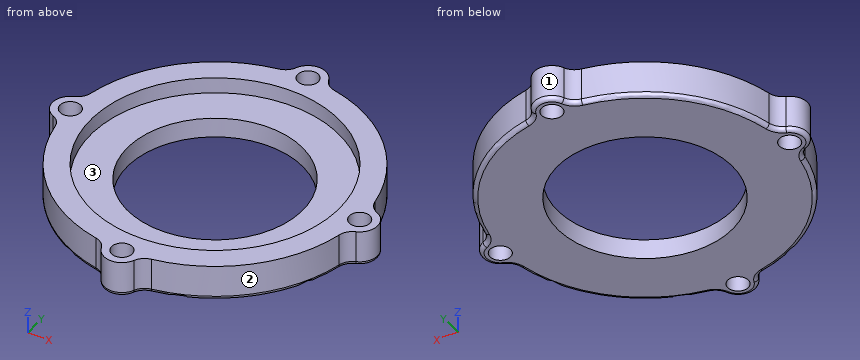
```python
from build123d import *

# Parameters (mm, degrees)
SKETCH_R      = 22
SKETCH_R_2    = 2.6
PAD_DEPTH     = 9
SKETCH001_R   = 31.2
SKETCH001_R_2 = 22
POCKET_DEPTH  = 4
FILLET_R      = 4
FILLET001_R   = 1


with BuildPart() as part:
    # Sketch → Pad (new body)
    with BuildSketch(Plane.XY):
        with BuildLine():
            ThreePointArc((-4.5, 36.725332), (-26.162951, 26.162951), (-36.725332, 4.5))
            Line((-37.000025, 4.5), (-36.725332, 4.5))
            ThreePointArc((-37.000025, 4.5), (-41.5, 0), (-37.000025, -4.5))
            Line((-37.000025, -4.5), (-36.725332, -4.5))
            ThreePointArc((-36.725332, -4.5), (-26.162951, -26.162951), (-4.5, -36.725332))
            Line((-4.5, -36.725332), (-4.5, -37))
            ThreePointArc((-4.5, -37), (0, -41.5), (4.5, -37.000001))
            Line((4.5, -36.725332), (4.5, -37.000001))
            ThreePointArc((4.5, -36.725332), (26.162951, -26.162951), (36.725332, -4.5))
            Line((36.725332, -4.5), (37.000003, -4.5))
            ThreePointArc((37.000003, -4.5), (41.5, 0), (37.000003, 4.5))
            Line((36.725332, 4.5), (37.000003, 4.5))
            ThreePointArc((36.725332, 4.5), (26.162951, 26.162951), (4.5, 36.725332))
            Line((4.5, 36.999999), (4.5, 36.725332))
            ThreePointArc((4.5, 36.999999), (1.1e-05, 41.5), (-4.5, 37.000021))
            Line((-4.5, 37.000021), (-4.5, 36.725332))
        make_face()
        Circle(SKETCH_R, mode=Mode.SUBTRACT)
        with Locations((0, 37)):
            Circle(SKETCH_R_2, mode=Mode.SUBTRACT)
        with Locations((0, -37)):
            Circle(SKETCH_R_2, mode=Mode.SUBTRACT)
        with Locations((-37, 0)):
            Circle(SKETCH_R_2, mode=Mode.SUBTRACT)
        with Locations((37, 0)):
            Circle(SKETCH_R_2, mode=Mode.SUBTRACT)
    extrude(amount=PAD_DEPTH)

    # Sketch001 → Pocket (cut)
    with BuildSketch(Plane.XY.offset(9)):
        Circle(SKETCH001_R)
        Circle(SKETCH001_R_2, mode=Mode.SUBTRACT)
    extrude(amount=-POCKET_DEPTH, mode=Mode.SUBTRACT)

    # Fillet
    fillet_edges = [part.edges().sort_by_distance(p)[0] for p in [
        (-36.725332, 4.5, 4.5),
        (-4.5, 36.725332, 4.5),
        (4.5, 36.725332, 4.5),
        (36.725332, 4.5, 4.5),
        (36.725332, -4.5, 4.5),
        (4.5, -36.725332, 4.5),
        (-4.5, -36.725332, 4.5),
        (-36.725332, -4.5, 4.5),
    ]]
    fillet(fillet_edges, radius=FILLET_R)

    # Fillet001
    fillet001_edges = [part.edges().sort_by_distance(p)[0] for p in [
        (-5.323601, 37.145487, 0),
        (-26.162951, 26.162951, 0),
        (0, 41.5, 0),
        (5.323601, 37.145487, 0),
        (26.162951, 26.162951, 0),
        (37.145487, 5.323601, 0),
        (41.5, 0, 0),
        (37.145487, -5.323601, 0),
        (26.162951, -26.162951, 0),
        (5.323601, -37.145487, 0),
        (0, -41.5, 0),
        (-5.323601, -37.145487, 0),
        (-26.162951, -26.162951, 0),
        (-37.145487, -5.323601, 0),
        (-41.5, 0, 0),
        (-37.145487, 5.323601, 0),
    ]]
    fillet(fillet001_edges, radius=FILLET001_R)


solid = part.part
```
Here's how the part is built. I have some questions about the finished solid (model axes, mm). Face numbers are marked on the shaded views. Round coordinates to 2 decimals unless told otherwise and drop trailing zeros. Order: outer loops, then holes, each group sorted by start corner. A loop starts at its lowest first (then second) coordinate and runs counter-clockwise, first axis right, second up. Notation, with made-up numbers: M 26.25,-23.5 L 76.25,-23.5 A25 cw 76.25,7.5 Z; hole C 29.25,3.25 d8. An arc over 180 degrees is marked long. Use CSV: the item, a comma, the result in double quotes.
1) If we mould it in two halves opening along Y, with no side actions, what happens to the marked faces 1, 2 and 3? For each: pulls with the +Y half, pulls with the -Y half, needs draft (parallel to the pull), parting line crosses it, or undercut.
Taken from the geometry:
face 1,"pulls with the +Y half"
face 2,"pulls with the -Y half"
face 3,"undercut"
2) I need wall thicknesses on line 1 along Y through (x, z) = (0, 4.5); line 2 along Y through (x, z) = (0, 6.8); line 3 along X through (y, z) = (2, 4.25). Which ranges of each line are inside material? Lowest first, please. Write a range as [from, to].
Taken from the geometry:
line 1,"[-41.5, -39.6], [-34.4, -22], [22, 34.4], [39.6, 41.5]"
line 2,"[-41.5, -39.6], [-34.4, -31.2], [31.2, 34.4], [39.6, 41.5]"
line 3,"[-41.03, -38.66], [-35.34, -21.91], [21.91, 35.34], [38.66, 41.03]"
3) I want a section at A-A (y = 0). List the corners of the cut face in (x, z) for me, then the cut area to 3 significant figures.
Taken from the geometry:
outline,"M -41.5,1 A1 ccw -40.5,0 L -39.6,0 L -39.6,9 L -41.5,9 Z; M -34.4,0 L -22,0 L -22,5 L -31.2,5 L -31.2,9 L -34.4,9 Z; M 22,0 L 34.4,0 L 34.4,9 L 31.2,9 L 31.2,5 L 22,5 Z; M 39.6,0 L 40.5,0 A1 ccw 41.5,1 L 41.5,9 L 39.6,9 Z"
area,"183 mm^2"
4) I want a section at B-B (z = 3.5). Count the separate pieces of the cut face and the enclosed holes in it, then the cut area to 3 significant figures.
Taken from the geometry:
separate pieces,"1"
enclosed holes,"5"
area,"2,830 mm^2"
5) I'm going to push flat-ended pins straight in: P1, Ø10, axis at x = 18, y = -8.5, coming from the +Z side; P2, Ø4, axis at y = -25.5, z = 3.5, coming from the +X side; P3, Ø2, axis at y = -10, z = 7, coming from the -X side. Where does each tip first touch, or does it pass through?
Taken from the geometry:
P1,"z = 5"
P2,"x = 28.58"
P3,"x = -35.89"
